Autodesk Inventor part; units mm, degrees
ref_plane "YZ Plane" through (0, 0, 0) normal (1, 0, 0) x (0, 1, 0)
ref_plane "XZ Plane" through (0, 0, 0) normal (0, 1, 0) x (-1, 0, 0)
ref_plane "XY Plane" through (0, 0, 0) normal (0, 0, 1) x (1, 0, 0)
sketch "Sketch1" plane through (0, 0, 0) normal (0, 0, 1) x (1, 0, 0)
  line L0 (-6, -6) -> (6, -6)
  line L1 (6, -6) -> (6, 6)
  line L2 (6, 6) -> (-6, 6)
  line L3 (-6, 6) -> (-6, -6)
  line L4 (-6, -6) -> (6, 6) construction
  line L5 (6, -6) -> (-6, 6) construction
  point P0 (0, 0)
  dimension "d0" = 12
  dimension "d1" = 12
extrude "Extrusion1" add sketch "Sketch1" along normal blind 6
sketch "Sketch2" plane through (0, 0, 0) normal (0, 0, -1) x (-1, 0, 0)
  circle A0 centre (0, 0) radius 4.1
  dimension "d4" = 8.2
extrude "Extrusion2" cut sketch "Sketch2" against normal blind 4
sketch "Sketch3" plane through (0, 0, 6) normal (0, 0, 1) x (1, 0, 0)
  circle A0 centre (0, 0) radius 1.9
  dimension "d7" = 3.8
extrude "Extrusion3" cut sketch "Sketch3" against normal blind 2
sketch "Sketch5" plane through (6, -6, 0) normal (1, 0, 0) x (0, 0, -1)
  line L0 (0, 12) -> (-6, 12)
  line L1 (-6, 0) -> (-6, 12)
  line L2 (-6, 12) -> (-6, 0)
  line L3 (-6, 0) -> (-20, -8.0829)
  line L4 (-20, -8.0829) -> (-20, -0.0829)
  line L5 (-20, -0.0829) -> (-6, 12)
  line L6 (0, 0) -> (0, 12)
  point P0 (0, 6)
  point P1 (0, 6)
  dimension "d13" = 120
  dimension "d14" = 20
  dimension "d15" = 8
extrude "Extrusion5" add sketch "Sketch5" against normal blind 2
sketch "Sketch6" plane through (6, -6, 0) normal (1, 0, 0) x (0, 0, -1)
  circle A0 centre (-17, -2.0829) radius 1.6
  line L0 (0, 0) -> (0, 12)
  line L1 (-6, 0) -> (-20, -8.0829)
  line L2 (-20, -0.0829) -> (-6, 12)
  point P0 (0, 6)
  point P1 (0, 6)
  dimension "d18" = 3.2
  dimension "d19" = 17
  dimension "d23" = 2
extrude "Extrusion6" cut sketch "Sketch6" against normal blind 2
mirror "Mirror1" about plane through (0, 0, 0) normal (1, 0, 0) of "Extrusion5", "Extrusion6"
fillet "Fillet1" radius 1 4 edges at (-6, 6, 3) (6, 6, 3) (-6, -6, 3) (6, -6, 3)
fillet "Fillet2" radius 0.5 1 edges at (4.1, 0, 4)
fillet "Fillet3" radius 0.5 2 edges at (-4, 0, 6) (4, 0, 6)
chamfer "Chamfer1" distance 3 angle 45 2 edges at (-5, -14.0829, 20) (5, -14.0829, 20)
fillet "Fillet4" radius 2 6 edges at (-5, -11.0829, 20) (-5, -12.5829, 17.4019) (-5, -6.0829, 20) (5, -6.0829, 20) (5, -11.0829, 20) (5, -12.5829, 17.4019)
properties part number "PrzegubDolny"
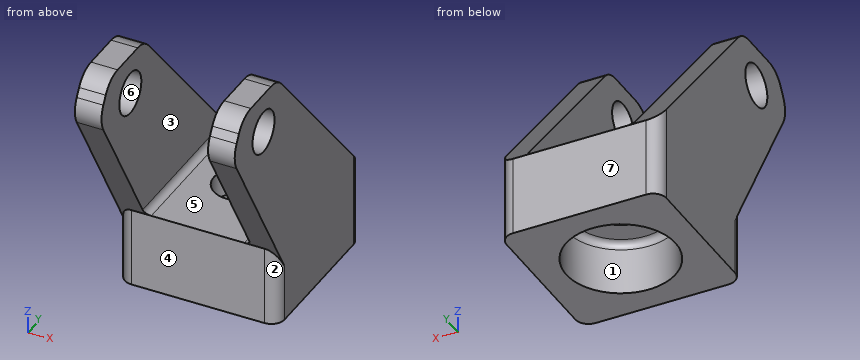
Model file for the job. Use its own axes, mm. Face numbers are marked on the shaded views. A direction names the side the tool comes from. Give positions to 0.01 mm unless a question says otherwise; leave off trailing zeros. Order: outer loops, then holes, each group sorted by start corner. A loop starts at its lowest first (then second) coordinate and runs counter-clockwise, first axis right, second up. Notation, with made-up numbers: M -36.5,31.5 L 12.5,31.5 A22 ccw 12.5,48.5 Z; hole C -10.5,14.5 d11. An arc over 180 degrees is marked long. Put each result on its own line as item: value. Start each with the question number.
(1) Band-saw the part on B-B on z = 12.25. Give the cut face in (x, y).
(2) Band-saw the part on D-D on z = 17. Give the cut face in (x, y).
(3) Tool access for the marked faces 1, 2, 3 and 4: list every direction of +Z, -Z, +X, -X, +Y, -Y with a clear straight run to the whole face (end or side of a thin tool).
(4) Drill centre lines: L1, parallel to X at y = 3.5, z = 7.75; L2, parallel to Z at x = 3, y = -4.5; L3, parallel to X at y = 3.5, z = 3.5. Where is each one in solid material? Low to high. Write a range as [from, to].
(5) Pull direction Z, two halves, no side cores. Call the marked faces 5, 6 and 7: released by +Z, released by -Z, zero draft, split by the parting line, or undercut.
(6) Band-saw the part on C-C on y = 0. Give the cut face in (x, z), then the cut area to 3 significant figures.
(7) Band-saw the part on A-A on x = 0. Give the cut face in (y, z).
(8) Pin check, flat tips, straight feed: pin 1 Ø5 at (x, y) = (0, 0) entering from +Z; pin 2 Ø3 at (y, z) = (-8.08, 17) entering from +X; pin 3 Ø6.5 at (x, z) = (-2, 4) entering from -Y; pin 4 Ø1 at (x, y) = (0, -2.5) entering from -Z. Stop position of each tip, or through.
Results below:
1. outline: M -6,-9.61 L -4,-9.61 L -4,0.61 L -6,0.61 Z; M 4,-9.61 L 6,-9.61 L 6,0.61 L 4,0.61 Z
2. outline: M -6,-12.23 L -4,-12.23 L -4,-9.68 L -6,-9.68 Z; M -6,-6.48 L -4,-6.48 L -4,-3.49 L -6,-3.49 Z; M 4,-12.23 L 6,-12.23 L 6,-9.68 L 4,-9.68 Z; M 4,-6.48 L 6,-6.48 L 6,-3.49 L 4,-3.49 Z
3. face 1: -Z
3. face 2: -Z, +X, -Y
3. face 3: +Z, +Y, -Y
3. face 4: -Z, +X, -X, -Y
4. L1: x = [-6, -4], [4, 6]
4. L2: z = [0, 6]
4. L3: x = [-6, -2.14], [2.14, 6]
5. face 5: released by +Z
5. face 6: undercut
5. face 7: zero draft
6. outline: M -6,0 L -4.1,0 L -4.1,3.5 A0.5 cw -3.6,4 L -1.9,4 L -1.9,6 L -3.5,6 A0.5 cw -4,6.5 L -4,12.95 L -6,12.95 Z; M 1.9,4 L 3.6,4 A0.5 cw 4.1,3.5 L 4.1,0 L 6,0 L 6,12.95 L 4,12.95 L 4,6.5 A0.5 cw 3.5,6 L 1.9,6 Z
6. area: 59.6 mm2
7. outline: M -6,0 L -4.1,0 L -4.1,3.5 A0.5 cw -3.6,4 L -1.9,4 L -1.9,6 L -6,6 Z; M 1.9,4 L 3.6,4 A0.5 cw 4.1,3.5 L 4.1,0 L 6,0 L 6,6 L 1.9,6 Z
8. pin 1: stops at z = 6
8. pin 2: passes through
8. pin 3: stops at y = -6.32
8. pin 4: stops at z = 4
